For this review, take the finished solid that the model builds, in its own axes (mm). Round coordinates to 2 decimals unless told otherwise and drop trailing zeros. Loops run counter-clockwise (first coordinate to the right, second up) from the corner with the lowest first, then second, coordinate; pieces in that order, holes last.
```python
from build123d import *

# Parameters (mm, degrees)
SKETCH1_R           = 2.413
SKETCH1_W           = 6.35
SKETCH1_H           = 6.35
SKETCH1_R_2         = 11.049
BOSS_EXTRUDE1_DEPTH = 6.35
BOSS_EXTRUDE4_DEPTH = 11.43
SKETCH7_R           = 2.413
CUT_EXTRUDE4_DEPTH  = 11.43
SKETCH8_R           = 2.413
CUT_EXTRUDE5_DEPTH  = 11.43
BOSS_EXTRUDE5_DEPTH = 11.43
SKETCH14_R          = 2.3114
CUT_EXTRUDE8_DEPTH  = 21.844
CUT_EXTRUDE9_DEPTH  = 21.844
FILLET3_R           = 1.27
FILLET4_R           = 5.08
FILLET5_R           = 7.62
FILLET6_START       = 3.433618276
FILLET6_DEPTH       = 6.8580001
FILLET6_START_2     = -2.219498454
FILLET6_2_DEPTH     = 12.636340452


with BuildPart() as part:
    # Sketch1 → Boss-Extrude1 (new body)
    with BuildSketch(Plane(origin=(0, 0, 0), x_dir=(1, 0, 0), z_dir=(0, 1, 0))):
        with BuildLine():
            ThreePointArc((-44.712520386, -1.790319958), (-41.464378908, -0.332372105), (-37.939187052, 0.166684391))
            Line((-37.939187052, 0.166684391), (-27.387614836, 0.166684391))
            Line((-27.387614836, 0.166684391), (-24.553673229, 0.166684391))
            ThreePointArc((-24.553673229, 0.166684391), (-19.165519557, -2.065161936), (-16.933673229, -7.453315609))
            Line((-16.933673229, -7.453315609), (-11.696120928, -38.563381903))
            ThreePointArc((-11.696120928, -38.563381903), (-9.102466616, -43.116571583), (-4.181867321, -44.918315609))
            Line((-4.181867321, -44.918315609), (2.671618376, -44.918315609))
            ThreePointArc((2.671618376, -44.918315609), (8.059772048, -42.686469281), (10.291618376, -37.298315609))
            Line((10.291618376, -37.298315609), (10.291618376, -36.576031258))
            Line((10.291618376, -36.576031258), (10.291618376, 31.928258006))
            Line((10.291618376, 31.928258006), (-62.328552859, 32.280391547))
            ThreePointArc((-62.328552859, 32.280391547), (-66.67527648, 36.888704376), (-68.255219526, 43.023387198))
            Line((-68.255219526, 43.023387198), (-68.255219526, 57.951684391))
            ThreePointArc((-68.255219526, 57.951684391), (-70.115091465, 62.441812452), (-74.605219526, 64.301684391))
            Line((-74.605219526, 64.301684391), (-103.180219526, 64.301684391))
            ThreePointArc((-103.180219526, 64.301684391), (-108.250679153, 60.73228976), (-111.435219526, 55.411684391))
            ThreePointArc((-111.435219526, 55.411684391), (-119.055219526, 9.691684391), (-111.435219526, -36.028315609))
            ThreePointArc((-111.435219526, -36.028315609), (-108.250679153, -41.348920977), (-103.180219526, -44.918315609))
            Line((-103.180219526, -44.918315609), (-74.605219526, -44.918315609))
            ThreePointArc((-74.605219526, -44.918315609), (-70.115091465, -43.058443669), (-68.255219526, -38.568315609))
            Line((-68.255219526, -38.568315609), (-68.255219526, -23.640018416))
            ThreePointArc((-68.255219526, -23.640018416), (-66.67527648, -17.505335593), (-62.328552859, -12.897022765))
            Line((-62.328552859, -12.897022765), (-44.712520386, -1.790319958))
        make_face()
        with Locations(Location((-103.180219526, -36.028315609, 0), (0, 0, 270))):
            Circle(SKETCH1_R, mode=Mode.SUBTRACT)
        with Locations(Location((-77.780219526, -36.028315609, 0), (0, 0, 270))):
            Circle(SKETCH1_R, mode=Mode.SUBTRACT)
        with Locations(Location((-77.780219526, -23.328315609, 0), (0, 0, 270))):
            Circle(SKETCH1_R, mode=Mode.SUBTRACT)
        with Locations((-77.780219526, -10.628315609)):
            Rectangle(SKETCH1_W, SKETCH1_H, mode=Mode.SUBTRACT)
        with Locations(Location((-1.580219526, -36.028315609, 0), (0, 0, 270))):
            Circle(SKETCH1_R, mode=Mode.SUBTRACT)
        with Locations(Location((-7.451232573, -7.453315609, 0), (0, 0, 270))):
            Circle(SKETCH1_R, mode=Mode.SUBTRACT)
        with Locations(Location((-111.435219526, 9.691684391, 0), (0, 0, 270))):
            Circle(SKETCH1_R, mode=Mode.SUBTRACT)
        with Locations((-77.780219526, 30.011684391)):
            Rectangle(SKETCH1_W, SKETCH1_H, mode=Mode.SUBTRACT)
        with Locations(Location((-103.180219526, 55.411684391, 0), (0, 0, 270))):
            Circle(SKETCH1_R, mode=Mode.SUBTRACT)
        with Locations(Location((-77.780219526, 42.711684391, 0), (0, 0, 270))):
            Circle(SKETCH1_R, mode=Mode.SUBTRACT)
        with Locations(Location((-77.780219526, 55.411684391, 0), (0, 0, 270))):
            Circle(SKETCH1_R, mode=Mode.SUBTRACT)
        with Locations((-45.551232573, 9.691684391)):
            Rectangle(SKETCH1_W, SKETCH1_H, mode=Mode.SUBTRACT)
        with Locations(Location((-7.451232573, 9.691684391, 0), (0, 0, 270))):
            Circle(SKETCH1_R_2, mode=Mode.SUBTRACT)
    extrude(amount=BOSS_EXTRUDE1_DEPTH)



with BuildPart() as body_2:
    # Sketch6 → Boss-Extrude4 (new body)
    with BuildSketch(Plane.XZ):
        Polygon((10.291618376, -2.219498454), (10.291618376, -16.715666773), (2.76121074, -24.725802919), (-1.31013754, -20.898288428), (4.703618376, -14.501423083), (4.703618376, -2.219498454), align=None)
    extrude(amount=BOSS_EXTRUDE4_DEPTH)

    # Sketch7 → Cut-Extrude4 (cut)
    with BuildSketch(Plane(origin=(13.805123423, 0, -12.978332071), x_dir=(-0.6849524859235093, 0, -0.7285877380434048), z_dir=(0.7285877380434048, 0, -0.6849524859235093))):
        with Locations((12.749560253, -5.715)):
            Circle(SKETCH7_R)
    extrude(amount=-CUT_EXTRUDE4_DEPTH, mode=Mode.SUBTRACT)

    # Sketch8 → Cut-Extrude5 (cut)
    with BuildSketch(Plane(origin=(10.291618376, 0, 0), x_dir=(0, 0, -1), z_dir=(1, 0, 0))):
        with Locations((9.007351169, -5.715)):
            Circle(SKETCH8_R)
    extrude(amount=-CUT_EXTRUDE5_DEPTH, mode=Mode.SUBTRACT)


with BuildPart() as part_1:
    add(part.part)

    add(body_2.part)  # Boss-Extrude5 merges body 2
    # Sketch13 → Boss-Extrude5 (add)
    with BuildSketch(Plane.XZ):
        Polygon((2.76121074, -24.725802919), (-12.621219973, -28.847512806), (-13.850827217, -24.258556099), (-1.31013754, -20.898288428), align=None)
    extrude(amount=BOSS_EXTRUDE5_DEPTH)

    # Sketch14 → Cut-Extrude8 (cut)
    with BuildSketch(Plane(origin=(6.366416777, 0, -23.759790873), x_dir=(-0.9659258262890685, 0, -0.2588190451025197), z_dir=(0.2588190451025197, 0, -0.9659258262890685))):
        with Locations((10.082383935, -5.719726248)):
            Circle(SKETCH14_R)
    extrude(amount=-CUT_EXTRUDE8_DEPTH, mode=Mode.SUBTRACT)

    # Sketch15 → Cut-Extrude9 (cut)
    with BuildSketch(Plane.XZ):
        Polygon((10.291618376, -16.715666773), (2.76121074, -24.725802919), (-24.752905313, -32.098188096), (10.291618376, -31.928258006), align=None)
    extrude(amount=-CUT_EXTRUDE9_DEPTH, mode=Mode.SUBTRACT)

    # Fillet3
    fillet3_edges = [part_1.edges().sort_by_distance(p)[0] for p in [
        (2.76121074, -2.54, -24.725802919),
        (-1.31013754, -5.715, -20.898288428),
        (-7.580482379, 0, -22.578422263),
        (4.703618376, 0, -8.360460768),
        (1.696740418, 0, -17.699855755),
        (4.703618376, -5.715, -14.501423083),
        (10.291618376, -2.54, -16.715666773),
    ]]
    fillet(fillet3_edges, radius=FILLET3_R)

    # Fillet4
    fillet4_edges = [part_1.edges().sort_by_distance(p)[0] for p in [
        (-13.400373689, 0, -25.939671553),
    ]]
    fillet(fillet4_edges, radius=FILLET4_R)

    # Fillet5
    fillet5_edges = [part_1.edges().sort_by_distance(p)[0] for p in [
        (-13.236023595, -11.43, -26.553034453),
    ]]
    fillet(fillet5_edges, radius=FILLET5_R)

    # Fillet6: read off the stored shape, not the designer's step
    # Fillet6 outline → Fillet6 (add)
    with BuildSketch(Plane.YZ.offset(FILLET6_START)):
        with BuildLine():
            Line((0, -2.219498454), (0, 10.416841998))
            ThreePointArc((0, 10.416841998), (-3.281427921, 1.897423003), (-11.43, -2.219498454))
            Line((-11.43, -2.219498454), (0, -2.219498454))
        make_face()
    extrude(amount=FILLET6_DEPTH)

    # Fillet6 2 outline → Fillet6 2 (cut)
    with BuildSketch(Plane.XY.offset(FILLET6_START_2)):
        with BuildLine():
            Line((4.703618377, -13), (4.703573688, -1.259346045))
            ThreePointArc((4.703573688, -1.259346045), (4.327869313, -0.368215513), (3.433618376, 0))
            Line((3.433618376, 0), (3.433618276, -13))
            Line((3.433618276, -13), (4.703618377, -13))
        make_face()
    extrude(amount=FILLET6_2_DEPTH, mode=Mode.SUBTRACT)


solid = part_1.part
```
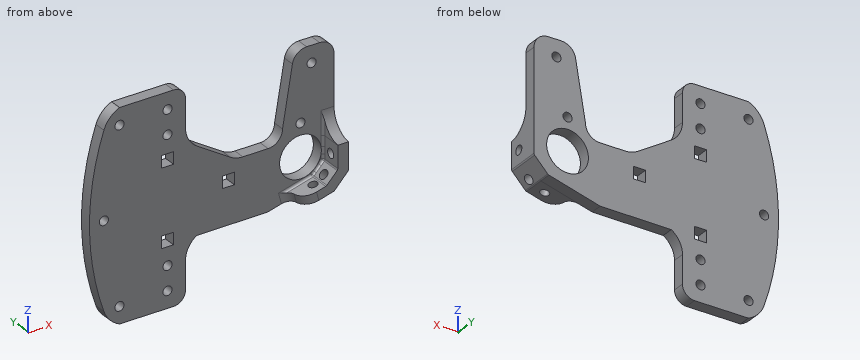
(1) Add section C-C (y = 2.75). Give the number of separate pieces and of enclosed holes in the cut face, plus the area to 3 significant figures.
(2) Add section A-A (z = 18). Give the boundary of the cut face in (x, y).
(3) Add section D-D (z = -48.5). Give the boundary of the cut face in (x, y).
(4) For L1, parallel to X at y = 1.5, z = 8; L2, parallel to X at y = 4.5, z = 13; L3, parallel to Y at x = -12, z = 20.5, list the stretches that pass through material, from the lowest coordinate up.
(5) Add section B-B (x = -47). Give the boundary of the cut face in (y, z).
(6) Insertion check: pin 1 Ø5.5 at (x, z) = (-77.78, -42.71) entering from -Y; pin 2 Ø1.9 at (x, y) = (-30, 3) entering from +Z; pin 3 Ø3 at (x, z) = (-77.78, 36.03) entering from -Y; pin 4 Ø3 at (y, z) = (3.5, 10) entering from -X. Each pin has a flat end and moves straight along its axis. Give the tip position at first contact, or say it passes through.
Outcome:
1. separate pieces: 1
1. enclosed holes: 13
1. area: 8,120 mm2
2. outline: (-116.31, 0) - (-66.93, 0) - (-66.93, 6.35) - (-116.31, 6.35) - close; (-15.16, 0) - (10.29, 0) - (10.29, 6.35) - (-15.16, 6.35) - close
3. outline: (-113.61, 0) - (-68.26, 0) - (-68.26, 6.35) - (-113.61, 6.35) - close
4. L1: x = -117.94 to -80.96, -74.61 to -54.56, -16.84 to -9.8, -5.1 to 10.29
4. L2: x = -117.22 to -80.96, -74.61 to -62.49, -16 to 10.29
4. L3: y = 0 to 6.35
5. outline: (0, -32.21) - (6.35, -32.21) - (6.35, -12.87) - (0, -12.87) - close; (0, -6.52) - (6.35, -6.52) - (6.35, 3.23) - (0, 3.23) - close
6. pin 1: stops at y = 0
6. pin 2: stops at z = -0.17
6. pin 3: passes through
6. pin 4: stops at x = -117.88
